from build123d import *

# Parameters (mm, degrees)
SKETCH1_R           = 3.68
BOSS_EXTRUDE1_DEPTH = 2
BOSS_EXTRUDE2_START = 3
SKETCH2_R           = 3.68
SKETCH2_R_2         = 2.375
BOSS_EXTRUDE2_DEPTH = 3
BOSS_EXTRUDE3_START = -2
BOSS_EXTRUDE3_DEPTH = 2
SKETCH7_R           = 1
CUT_EXTRUDE4_DEPTH  = 2
SKETCH8_R           = 2
CUT_EXTRUDE6_DEPTH  = 1.5


with BuildPart() as part:
    # Sketch1 → Boss-Extrude1 (new body)
    with BuildSketch(Plane(origin=(0, 0, 0), x_dir=(1, 0, 0), z_dir=(0, 1, 0))):
        with Locations(Location((0, 0, 0), (0, 0, 270))):
            Circle(SKETCH1_R)
    extrude(amount=-BOSS_EXTRUDE1_DEPTH)

    # Sketch2 → Boss-Extrude2 (add)
    with BuildSketch(Plane(origin=(0, 0, 0), x_dir=(1, 0, 0), z_dir=(0, 1, 0)).offset(BOSS_EXTRUDE2_START)):
        with Locations(Location((0, 0, 0), (0, 0, 270))):
            Circle(SKETCH2_R)
        with Locations(Location((0, 0, 0), (0, 0, 270))):
            Circle(SKETCH2_R_2, mode=Mode.SUBTRACT)
    extrude(amount=-BOSS_EXTRUDE2_DEPTH)

    # Sketch6 → Boss-Extrude3 (add)
    with BuildSketch(Plane.XZ.offset(2).offset(BOSS_EXTRUDE3_START)):
        with BuildLine():
            Line((0, -3.68), (-20, -3.68))
            ThreePointArc((-20, -3.68), (-23.68, 0), (-20, 3.68))
            Line((-20, 3.68), (0, 3.68))
            ThreePointArc((0, 3.68), (3.68, 0), (0, -3.68))
        make_face()
    extrude(amount=BOSS_EXTRUDE3_DEPTH)

    # Sketch7 → Cut-Extrude4 (cut)
    with BuildSketch(Plane.XZ.offset(2)):
        with Locations(Location((0, 0, 0), (0, 0, 270))):
            Circle(SKETCH7_R)
        with Locations(Location((-20, 0, 0), (0, 0, 270))):
            Circle(SKETCH7_R)
    extrude(amount=-CUT_EXTRUDE4_DEPTH, mode=Mode.SUBTRACT)

    # Sketch8 → Cut-Extrude6 (cut)
    with BuildSketch(Plane.XZ.offset(2)):
        with Locations(Location((0, 0, 0), (0, 0, 270))):
            Circle(SKETCH8_R)
    extrude(amount=-CUT_EXTRUDE6_DEPTH, mode=Mode.SUBTRACT)


solid = part.part
Work out the finished part from the listing and answer in its coordinate system (mm). A direction names the side the tool comes from. Give positions to 0.01 mm unless a question says otherwise; leave off trailing zeros. Loops run counter-clockwise (first coordinate to the right, second up) from the corner with the lowest first, then second, coordinate; pieces in that order, holes last. Notation, with made-up numbers: (-19.75, 8.25) -> (27.25, 8.25) arc R24 ccw to (27.25, 44.25) -> close; hole circle Ø9 at (49, 78.25). An arc over 180 degrees is marked (long way). Use a Markdown table: item, result. Add a question column.
1) Consider line 1 along X through (y, z) = (-0.1, 0); line 2 along X through (y, z) = (-1.5, 0); line 3 along Y through (x, z) = (-12, 2.25). Determine where each line is inside the solid, lowest interval first.
2) Each of these flat-tipped pins is pushed along its axis until it touches: P1, Ø1.5, axis at y = 1.5, z = 3, coming from the -X side; P2, Ø2, axis at y = 1.5, z = -2, coming from the -X side; P3, Ø1.8, axis at x = -20, z = 0, coming from the +Y side; P4, Ø1.4, axis at x = -0.5, z = 0, coming from the +Y side. Where does it stop, or does it pass through?
3) Which of the six approach directions +Z, -Z, +X, -X, +Y, -Y give full straight-line access (tool end or side, diameter ignored) to faces 4 (the flat face through (-1, -0.5, -1)), 5 (the cylindrical face through (-1.45, 1.52, -1.88)), 6 (the cylindrical face through (-21, -1, 0))?
4) The part is cut by section D-D, the plane y = 1.25. Determine the outline of the cut face in (x, z) (3 decimals), plus the area to 3 significant figures.
5) For a pull along X with two mould halves and no side action, classify faces 1 (the cylindrical face through (3.65, 1.09, -0.48)), 2 (the cylindrical face through (-2, -1, 0)), 3 (the flat face through (-10, -1, 3.68)) as +X half, -X half, draft (parallel to the pull), parting line (faces both ways), or undercut.
6) The part is cut by section C-C, the plane x = -1.5. Determine the outline of the cut face in (y, z).
7) The part is cut by section B-B, the plane x = -20.25. Determine the outline of the cut face in (y, z), plus the area to 3 significant figures.
8) The part is cut by section A-A, the plane z = 0. Determine the outline of the cut face in (x, y) (3 decimals).
Reported:
| question | item | result |
|---|---|---|
| 1 | line 1 | x = -23.68 to -21, -19 to -1, 1 to 3.68 |
| 1 | line 2 | x = -23.68 to -21, -19 to -2, 2 to 3.68 |
| 1 | line 3 | y = -2 to 0 |
| 2 | P1 | stops at x = -2.91 |
| 2 | P2 | stops at x = -3.54 |
| 2 | P3 | passes through |
| 2 | P4 | stops at y = 0 |
| 3 | face 4 | -Y |
| 3 | face 5 | +Y |
| 3 | face 6 | +Y, -Y |
| 4 | outline | circle Ø7.36 at (0, 0); hole circle Ø4.75 at (0, 0) |
| 4 | area | 24.8 mm^2 |
| 5 | face 1 | parting line |
| 5 | face 2 | undercut |
| 5 | face 3 | draft |
| 6 | outline | (-2, -3.68) -> (0, -3.68) -> (0, -3.36) -> (3, -3.36) -> (3, -1.84) -> (0, -1.84) -> (0, 1.84) -> (3, 1.84) -> (3, 3.36) -> (0, 3.36) -> (0, 3.68) -> (-2, 3.68) -> (-2, 1.32) -> (-0.5, 1.32) -> (-0.5, -1.32) -> (-2, -1.32) -> close |
| 7 | outline | (-2, -3.67) -> (0, -3.67) -> (0, -0.97) -> (-2, -0.97) -> close; (-2, 0.97) -> (0, 0.97) -> (0, 3.67) -> (-2, 3.67) -> close |
| 7 | area | 10.8 mm^2 |
| 8 | outline | (-23.68, -2) -> (-21, -2) -> (-21, 0) -> (-23.68, 0) -> close; (-19, -2) -> (-2, -2) -> (-2, -0.5) -> (-1, -0.5) -> (-1, 0) -> (-2.375, 0) -> (-2.375, 3) -> (-3.68, 3) -> (-3.68, 0) -> (-19, 0) -> close; (1, -0.5) -> (2, -0.5) -> (2, -2) -> (3.68, -2) -> (3.68, 3) -> (2.375, 3) -> (2.375, 0) -> (1, 0) -> close |
